Here's how the part is built. I have some questions about the finished solid (model axes, mm). A direction names the side the tool comes from. Give positions to 0.01 mm unless a question says otherwise; leave off trailing zeros. Loops run counter-clockwise (first coordinate to the right, second up) from the corner with the lowest first, then second, coordinate; pieces in that order, holes last.
Q1. We'd pull the mould along Z, two halves only. Please class faces 5 (the face through (3, 56, -105.284)), 6 (the face through (3, 48.26, -77)), 7 (the face through (3, 17, 0)): +Z half, -Z half, draft (parallel to the pull), parting line (faces both ways), or undercut.
Q2. Will these pins go through, and if not, where does the flat tip stop? P1, Ø1.3, axis at x = 4.5, y = 48, coming from the +Z side; P2, Ø2.5, axis at x = 3, y = 2.5, coming from the -Z side.
Q3. If we section it at D-D (y = 60): Please give me the cut outline in (x, z).
Q4. If we section it at A-A (z = -57.5): Please give me the cut outline in (x, y).
Q5. I need wall thicknesses on line 1 (Y direction, x = 4, z = -74.5); line 2 (Y direction, x = 5.5, z = -93); line 3 (Z direction, x = 2.25, y = 51.5). Which ranges of each line are inside material? Lowest first, please.
Q6. If we section it at C-C (z = -89.5): Please give me the cut outline in (x, y).
Q7. For faces 1 (the face through (3, 2, -93.98)), 2 (the face through (3, 46.672, -76)), 3 (the face through (3, 50, -6.35)), 4 (the face through (3.131, 39.048, -91.343)), which set-ups out of +Z, -Z, +X, -X, +Y, -Y let a thin tool reach every point of the face, with its end or its side?
Autodesk Inventor part; units mm, degrees
ref_plane "YZ Plane" through (0, 0, 0) normal (1, 0, 0) x (0, 1, 0)
ref_plane "XZ Plane" through (0, 0, 0) normal (0, 1, 0) x (-1, 0, 0)
ref_plane "XY Plane" through (0, 0, 0) normal (0, 0, 1) x (1, 0, 0)
sketch "Sketch1" plane through (0, 0, 0) normal (1, 0, 0) x (0, 1, 0)
  line L0 (0, 0) -> (0, -93.98)
  line L1 (0, -93.98) -> (3.175, -93.98)
  line L2 (3.175, -93.98) -> (31.2212, -77.7875)
  line L3 (31.2212, -77.7875) -> (47.0962, -105.2838)
  line L4 (47.0962, -105.2838) -> (66.04, -105.2838)
  line L5 (66.04, -105.2838) -> (66.04, -6.35)
  line L6 (34.29, 0) -> (0, 0)
  line L7 (48.26, -54.61) -> (46.6725, -54.61)
  line L8 (46.6725, -54.61) -> (46.6725, -97.79)
  line L9 (46.6725, -97.79) -> (48.26, -97.79)
  line L10 (48.26, -97.79) -> (48.26, -54.61)
  line L11 (66.04, -6.35) -> (34.29, -6.35)
  line L12 (34.29, -6.35) -> (34.29, 0)
  dimension "d2" = 31.75
  dimension "d4" = 30
  dimension "d6" = 66.04
  dimension "d7" = 93.98
  dimension "d8" = 32.385
  dimension "d9" = 3.175
  dimension "d10" = 43.18
  dimension "d11" = 1.5875
  dimension "d13" = 54.61
  dimension "d16" = 6.35
  dimension "d17" = 31.75
  dimension "d18" = 48.26
extrude "Extrusion1" add sketch "Sketch1" along normal blind 6.35
properties part number "chute_wall"
Check sheet entries:
1. face 5: -Z half
1. face 6: undercut
1. face 7: +Z half
2. P1: stops at z = -6.35
2. P2: stops at z = -93.98
3. outline: (0, -105.28) - (6.35, -105.28) - (6.35, -6.35) - (0, -6.35) - close
4. outline: (0, 0) - (6.35, 0) - (6.35, 46.67) - (0, 46.67) - close; (0, 48.26) - (6.35, 48.26) - (6.35, 66.04) - (0, 66.04) - close
5. line 1: y = 0 to 46.67, 48.26 to 66.04
5. line 2: y = 0 to 4.87, 40 to 46.67, 48.26 to 66.04
5. line 3: z = -105.28 to -6.35
6. outline: (0, 0) - (6.35, 0) - (6.35, 10.93) - (0, 10.93) - close; (0, 37.98) - (6.35, 37.98) - (6.35, 46.67) - (0, 46.67) - close; (0, 48.26) - (6.35, 48.26) - (6.35, 66.04) - (0, 66.04) - close
7. face 1: -Z, +X, -X, -Y
7. face 2: +X, -X
7. face 3: +Z, +X, -X, +Y
7. face 4: -Z, +X, -X
